```python
from build123d import *

# Parameters (mm, degrees)
EXTRUDE_2_DEPTH     = 14
SKETCH_2_R          = 2.75
CUT_EXTRUDE_1_DEPTH = 37.813584449


with BuildPart() as part:
    # 草图1 → 凸台-拉伸2 (new body)
    with BuildSketch(Plane.XY):
        with BuildLine():
            Line((21, -20), (-21, -20))
            Line((-21, -20), (-21, -14))
            Line((-21, -14), (-9, -14))
            Line((-9, -14), (-9, 12.8))
            Line((-9, 12.8), (-0.438791817, 12.8))
            Line((-0.438791817, 12.8), (-0.438791817, 3.975859874))
            ThreePointArc((-0.438791817, 3.975859874), (0, -4), (0.438791817, 3.975859874))
            Line((0.438791817, 3.975859874), (0.438791817, 12.8))
            Line((0.438791817, 12.8), (9, 12.8))
            Line((9, 12.8), (9, -14))
            Line((9, -14), (21, -14))
            Line((21, -14), (21, -20))
        make_face()
    extrude(amount=EXTRUDE_2_DEPTH)

    # 草图2 → 切除-拉伸1 (cut, through all)
    with BuildSketch(Plane(origin=(0, -14, 0), x_dir=(1, 0, 0), z_dir=(0, 1, 0))):
        with Locations(Location((-16, -7, 0), (0, 0, 270))):
            Circle(SKETCH_2_R)
        with Locations(Location((16, -7, 0), (0, 0, 270))):
            Circle(SKETCH_2_R)
    extrude(amount=-CUT_EXTRUDE_1_DEPTH, mode=Mode.SUBTRACT)


solid = part.part
```
Geometry check sheet. Reference: the model listing, model coordinates, mm. A direction names the side the tool comes from. Coordinates: 2 decimals unless noted, no trailing zeros. Loops run counter-clockwise (first coordinate to the right, second up) from the corner with the lowest first, then second, coordinate; pieces in that order, holes last. Notation, with made-up numbers: (75.25, 10) -> (99.25, 10) arc R24 cw to (99.25, 38) -> close; hole circle Ø1 at (-22.5, 40). An arc over 180 degrees is marked (long way). Put each result on its own line as item: value.
1) Cross-section at D-D on z = 2.5. Record the boundary of the cut face in (x, y), plus the area to 3 significant figures.
Result set:
outline: (-21, -20) -> (21, -20) -> (21, -14) -> (9, -14) -> (9, 12.8) -> (0.44, 12.8) -> (0.44, 3.98) arc R4 cw (long way) to (-0.44, 3.98) -> (-0.44, 12.8) -> (-9, 12.8) -> (-9, -14) -> (-21, -14) -> close
area: 676 mm^2
2) Cross-section at B-B on z = 7. Record the boundary of the cut face in (x, y).
Result set:
outline: (-21, -20) -> (-18.75, -20) -> (-18.75, -14) -> (-21, -14) -> close; (-13.25, -20) -> (13.25, -20) -> (13.25, -14) -> (9, -14) -> (9, 12.8) -> (0.44, 12.8) -> (0.44, 3.98) arc R4 cw (long way) to (-0.44, 3.98) -> (-0.44, 12.8) -> (-9, 12.8) -> (-9, -14) -> (-13.25, -14) -> close; (18.75, -20) -> (21, -20) -> (21, -14) -> (18.75, -14) -> close
3) Gauge pin test, flat ends, axial feed: pin 1 Ø4 at (x, y) = (-12.5, 5.5) entering from -Z; pin 2 Ø2.5 at (y, z) = (9.5, 6.5) entering from +X; pin 3 Ø3.5 at (x, z) = (13, 7) entering from +Y; pin 4 Ø2.5 at (y, z) = (7.5, 5.5) entering from -X. Record the tip position at first contact, or that the pin passes through.
Result set:
pin 1: passes through
pin 2: stops at x = 9
pin 3: stops at y = -14
pin 4: stops at x = -9
4) Release check for a two-part mould opening along X. For faces 6 (the flat face through (-5, 12.8, 7)), 7 (the flat face through (0.439, 8, 7)), 8 (the flat face through (-9, -1, 7)) record: released by +X, released by -X, zero draft, split by the parting line, or undercut.
Result set:
face 6: zero draft
face 7: undercut
face 8: released by -X
5) Cross-section at A-A on x = 16. Record the boundary of the cut face in (y, z).
Result set:
outline: (-20, 0) -> (-14, 0) -> (-14, 4.25) -> (-20, 4.25) -> close; (-20, 9.75) -> (-14, 9.75) -> (-14, 14) -> (-20, 14) -> close
6) Thickness scan on line 1 (X direction, y = -16.45, z = 7); line 2 (X direction, y = 0, z = 4.5); line 3 (X direction, y = 11.5, z = 9). Record the ranges inside material, lowest first.
Result set:
line 1: x = -21 to -18.75, -13.25 to 13.25, 18.75 to 21
line 2: x = -9 to -4, 4 to 9
line 3: x = -9 to -0.44, 0.44 to 9
7) Cross-section at C-C on y = -3. Record the boundary of the cut face in (x, z), plus the area to 3 significant figures.
Result set:
outline: (-9, 0) -> (-2.65, 0) -> (-2.65, 14) -> (-9, 14) -> close; (2.65, 0) -> (9, 0) -> (9, 14) -> (2.65, 14) -> close
area: 178 mm^2
8) Tool access check on faces 1 (the flat face through (13.6, -14, 5.3)), 2 (the cylindrical face through (18.727, -16.958, 6.642)), 3 (the flat face through (0, -20, 7)), 4 (the flat face through (-0.439, 8, 7)), 5 (the flat face through (-12, -14, 7)). Record the directions out of +Z, -Z, +X, -X, +Y, -Y that give a thin tool (end or side, any length) a straight path to the whole face; none if there is none.
Result set:
face 1: +Z, -Z, +X, +Y
face 2: +Y, -Y
face 3: +Z, -Z, +X, -X, -Y
face 4: +Z, -Z, +Y
face 5: +Z, -Z, -X, +Y
